from build123d import *

# Parameters (mm, degrees)
SKETCH1_W           = 74
SKETCH1_H           = 74
BOSS_EXTRUDE1_DEPTH = 31
SKETCH2_W           = 26.106590286
SKETCH2_H           = 5.588637075
BOSS_EXTRUDE2_DEPTH = 12.7


with BuildPart() as part:
    # Sketch1 → Boss-Extrude1 (new body)
    with BuildSketch(Plane(origin=(0, 0, 0), x_dir=(1, 0, 0), z_dir=(0, 1, 0))):
        with Locations((37, 37)):
            Rectangle(SKETCH1_W, SKETCH1_H)
    extrude(amount=BOSS_EXTRUDE1_DEPTH)

    # Sketch2 → Boss-Extrude2 (add)
    with BuildSketch(Plane.XY):
        with Locations((37, 2.794318538)):
            Rectangle(SKETCH2_W, SKETCH2_H)
    extrude(amount=BOSS_EXTRUDE2_DEPTH)


solid = part.part
Geometry check sheet. Reference: the model listing, model coordinates, mm. A direction names the side the tool comes from. Coordinates: 2 decimals unless noted, no trailing zeros. Order: outer loops, then holes, each group sorted by start corner. A loop starts at its lowest first (then second) coordinate and runs counter-clockwise, first axis right, second up. Notation, with made-up numbers: (32.5, 29.25) -> (72.5, 29.25) arc R19 cw to (72.5, 42.25) -> close; hole circle Ø4 at (-18.5, 78.25). An arc over 180 degrees is marked (long way). Use a Markdown table: item, result. Add a question column.
1. Set-up check for faces 1 (the face through (36, 0, -31)), 2 (the face through (50.053, 3, 6)), 3 (the face through (23.947, 3, 6)), 4 (the face through (37, 5.589, 6)), 5 (the face through (74, 15, -36)): record each of +Z, -Z, +X, -X, +Y, -Y from which the full face is reachable in a straight line by a thin tool's end or side.
2. Cross-section at C-C (x = 9.5). Enter the section's corners in (y, z), and give its area (3 significant figures).
3. Go/stop test with flat-tipped pins: pin 1 Ø1.7 at (y, z) = (2, 5) entering from +X; pin 2 Ø3 at (x, y) = (18.5, 3.5) entering from +Z; pin 3 Ø6 at (y, z) = (2.5, 7.5) entering from -X. Record where each tip stops, or that it passes through.
4. Cross-section at B-B (y = 21). Enter the section's corners in (x, z), and give its area (3 significant figures).
5. Cross-section at A-A (x = 34.5). Enter the section's corners in (y, z), and give its area (3 significant figures).
6. Material ranges on L1, parallel to Z at x = 8.5, y = 21, recorded low to high.
Filled sheet:
| question | item | result |
|---|---|---|
| 1 | face 1 | +Z, -Z, +X, -X, -Y |
| 1 | face 2 | +Z, +X, +Y, -Y |
| 1 | face 3 | +Z, -X, +Y, -Y |
| 1 | face 4 | +Z, +X, -X, +Y |
| 1 | face 5 | +Z, -Z, +X, +Y, -Y |
| 2 | outline | (0, -74) -> (31, -74) -> (31, 0) -> (0, 0) -> close |
| 2 | area | 2,290 mm2 |
| 3 | pin 1 | x = 50.05 |
| 3 | pin 2 | z = 0 |
| 3 | pin 3 | x = 23.95 |
| 4 | outline | (0, -74) -> (74, -74) -> (74, 0) -> (0, 0) -> close |
| 4 | area | 5,480 mm2 |
| 5 | outline | (0, -74) -> (31, -74) -> (31, 0) -> (5.59, 0) -> (5.59, 12.7) -> (0, 12.7) -> close |
| 5 | area | 2,360 mm2 |
| 6 | L1 | -74 to 0 |
